Input: dimensioned drawing with shaded views. Units: mm. Origin: part minimum x, y, z. A direction names the side the tool comes from. Give positions to 0.01 mm unless a question says otherwise; leave off trailing zeros. Write each loop counter-clockwise with the first axis right and the second up, starting at its lowest first coordinate (ties: lowest second). Pieces come first, ordered by that corner, then holes. Notation, with made-up numbers: M -4.75,33.5 L 4.25,33.5 A26 ccw 4.25,59.5 Z; hole C 14.5,41.5 d4. An arc over 180 degrees is marked long. Answer as a JSON object with one key per item and string values.
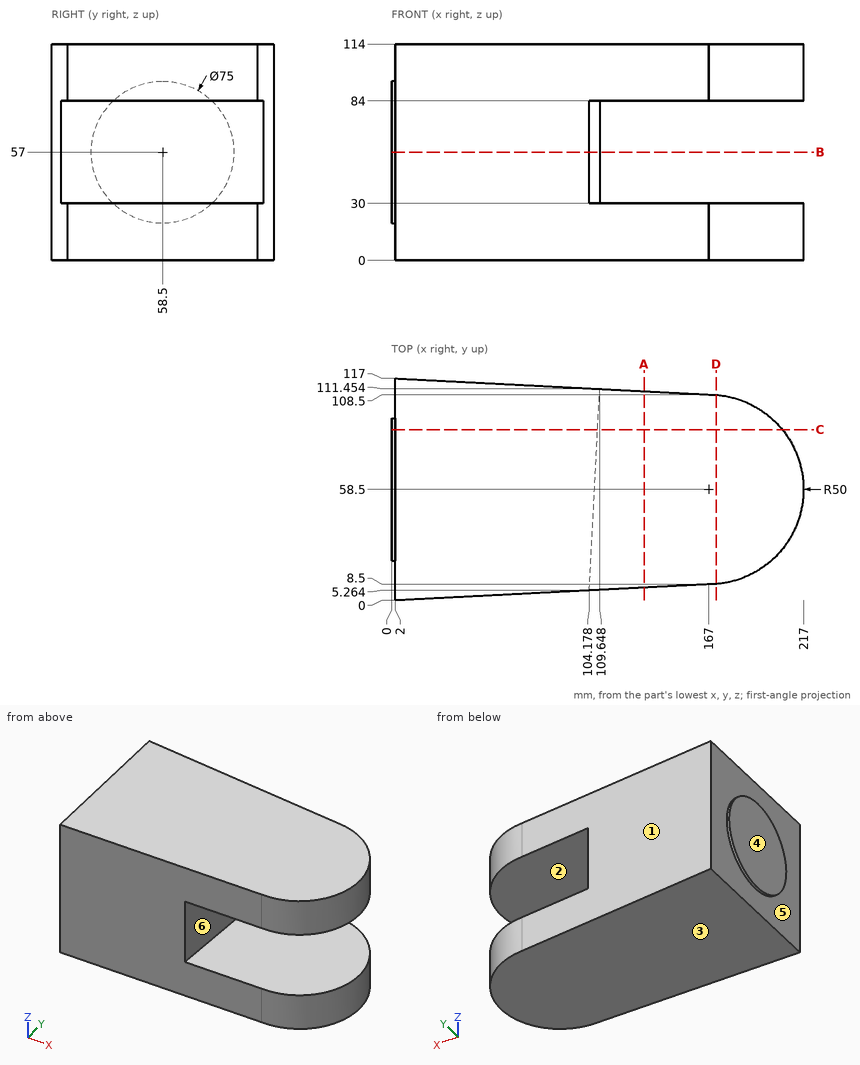
1) Cut plane A-A on x = 133. Return loops of the section in (y, z), and give its area (3 significant figures).
Geometry check:
{"outline": "M 6.75,0 L 110.25,0 L 110.25,30 L 6.75,30 Z; M 6.75,84 L 110.25,84 L 110.25,114 L 6.75,114 Z", "area": "6,210 mm2"}
2) Pull-direction query (Z, two-part tool) for the marked faces 1, 2 and 3; classes: pulls with the +Z half, pulls with the -Z half, needs draft (parallel to the pull), parting line crosses it, or undercut.
Geometry check:
{"face 1": "needs draft", "face 2": "undercut", "face 3": "pulls with the -Z half"}
3) Contact query for flat-ended pins moving along their axis: P1, Ø10, axis at y = 45.5, z = 67.5, coming from the +X side; P2, Ø1.5, axis at y = 38, z = 16, coming from the +X side (1 decimal); P3, Ø10, axis at y = 78.5, z = 67, coming from the +X side; P4, Ø8, axis at x = 151.5, z = 79.5, coming from the -Y side. Output: stop coordinate, or through.
Geometry check:
{"P1": "stops at x = 106.51", "P2": "stops at x = 212.9", "P3": "stops at x = 108.21", "P4": "passes through"}
4) Line query: line 1 (Z direction, x = 125, y = 10); line 2 (Y direction, x = 72, z = 86.5) (1 decimal); line 3 (X direction, y = 25, z = 82.5) (1 decimal). Output: solid intervals per line, ascending. Write a range as from..to.
Geometry check:
{"line 1": "z = 0..30, 84..114", "line 2": "y = 3.6..113.4", "line 3": "x = 2..105.2"}
5) Cut plane B-B on z = 57. Return loops of the section in (x, y) (1 decimal).
Geometry check:
{"outline": "M 0,21 L 2,21 L 2,0 L 104.2,5.3 L 109.6,111.5 L 2,117 L 2,96 L 0,96 Z"}
6) Cut plane D-D on x = 171. Return loops of the section in (y, z), and give its area (3 significant figures).
Geometry check:
{"outline": "M 8.66,0 L 108.34,0 L 108.34,30 L 8.66,30 Z; M 8.66,84 L 108.34,84 L 108.34,114 L 8.66,114 Z", "area": "5,980 mm2"}
7) Set-up query: the marked faces 4, 5 and 6. Return all of +Z, -Z, +X, -X, +Y, -Y with unobstructed straight access to the full face (end or side cutting, diameter ignored); none if empty.
Geometry check:
{"face 4": "+Z, -Z, -X, +Y, -Y", "face 5": "-X", "face 6": "+X, -Y"}
8) Cut plane C-C on y = 90. Return loops of the section in (x, z).
Geometry check:
{"outline": "M 0,36.65 L 2,36.65 L 2,0 L 205.83,0 L 205.83,30 L 108.54,30 L 108.54,84 L 205.83,84 L 205.83,114 L 2,114 L 2,77.35 L 0,77.35 Z"}
